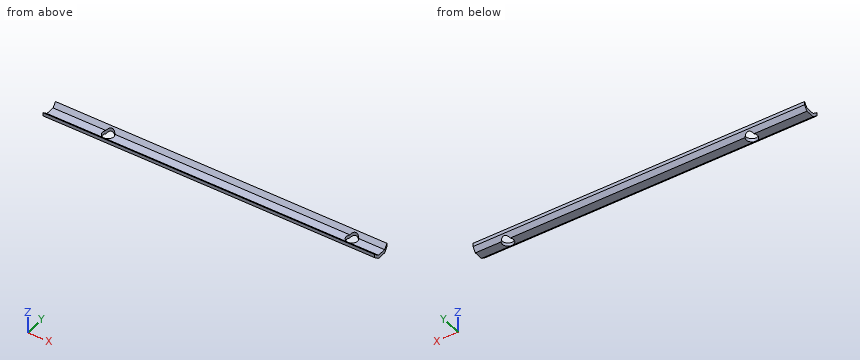
from build123d import *

# Parameters (mm, degrees)
MAIN_BODY_EXTRUDE_DEPTH       = 147.5
CROSS_BOLT_BORE_SKETCH_R      = 2.5
CROSS_BOLT_BORE_EXTRUDE_DEPTH = 148.758248501


with BuildPart() as part:
    # Main Body Sketch → Main Body Extrude (new body)
    with BuildSketch(Plane(origin=(0, 0, 0), x_dir=(0, 0, -1), z_dir=(1, 0, 0))):
        Polygon((0, 0), (2, -1.5), (2, -5.5), (0, -8), (1.5, -8), (3.5, -5.5), (3.5, -1.5), (1.5, 0), align=None)
    extrude(amount=-MAIN_BODY_EXTRUDE_DEPTH)

    # Cross Bolt Bore Sketch → Cross Bolt Bore Extrude (cut, through all)
    with BuildSketch(Plane(origin=(0, 0, -3.5), x_dir=(-1, 0, 0), z_dir=(0, 0, -1))):
        with Locations(Location((13.5, -3, 0), (0, 0, 143.130102354))):
            Circle(CROSS_BOLT_BORE_SKETCH_R)
        with Locations(Location((122, -3, 0), (0, 0, 36.869897646))):
            Circle(CROSS_BOLT_BORE_SKETCH_R)
    extrude(amount=-CROSS_BOLT_BORE_EXTRUDE_DEPTH, mode=Mode.SUBTRACT)


solid = part.part
CAD build for the part. Positions are in the model's coordinates, mm. Give positions to 0.01 mm unless a question says otherwise; leave off trailing zeros. Order: outer loops, then holes, each group sorted by start corner. A loop starts at its lowest first (then second) coordinate and runs counter-clockwise, first axis right, second up. Notation, with made-up numbers: (42, -20.75) - (101, -20.75) arc R13 ccw to (101, 4.25) - close; hole circle Ø4 at (70, -8.5). An arc over 180 degrees is marked (long way). Answer in a Markdown table with one row per item.
1. Probe probe 1 along X at (y, z) = (-3, -2.3); probe 2 along X at (y, z) = (-4, -2.8); probe 3 along Z at (x, y) = (-119, -3.75). List the from-to ranges inside material, lowest first. Write a range as [from, to].
Data:
| item | result |
|---|---|
| probe 1 | x = [-147.5, -124.5], [-119.5, -16], [-11, 0] |
| probe 2 | x = [-147.5, -124.29], [-119.71, -15.79], [-11.21, 0] |
| probe 3 | z = [-3.5, -2] |
2. Flat gauge pins, fed straight in: pin 1 (2 mm diameter, centred on x = -132, y = -3, fed in from +Z); pin 2 (4 mm diameter, centred on x = -13.5, y = -3, fed in from -Z). Where does each tip first touch, or does it go through?
Data:
| item | result |
|---|---|
| pin 1 | stops at z = -2 |
| pin 2 | passes through |
3. Saw through at B-B, the plane x = -71.5. Give the cut face in (y, z).
Data:
| item | result |
|---|---|
| outline | (-8, -1.5) - (-5.5, -3.5) - (-1.5, -3.5) - (0, -1.5) - (0, 0) - (-1.5, -2) - (-5.5, -2) - (-8, 0) - close |
4. Saw through at A-A, the plane y = -3. Give the cut face in (x, z).
Data:
| item | result |
|---|---|
| outline | (-147.5, -3.5) - (-124.5, -3.5) - (-124.5, -2) - (-147.5, -2) - close; (-119.5, -3.5) - (-16, -3.5) - (-16, -2) - (-119.5, -2) - close; (-11, -3.5) - (0, -3.5) - (0, -2) - (-11, -2) - close |
